Input: part model. Units: mm. Frame: model coordinates. Face numbers are marked on the shaded views. A direction names the side the tool comes from. Round coordinates to 2 decimals unless told otherwise and drop trailing zeros. Loops run counter-clockwise (first coordinate to the right, second up) from the corner with the lowest first, then second, coordinate; pieces in that order, holes last. Notation, with made-up numbers: M 38,44 L 47,44 A22 cw 47,79 Z; hole C 37,33.25 d5. An arc over 180 degrees is marked long. Use one line per item in the form item = value. Start each with the question number.
Q1. Ray query, line 1 along X through (y, z) = (0, 2.95); line 2 along X through (y, z) = (0, 1.85); line 3 along Y through (x, z) = (110, 3.9). Return the intervals inside material, ascending.
Q2. Section query C-C, the plane z = 5. Output: boundary loops of the cut face in (x, y).
Q3. Access query for the marked faces 5 and 6. Directions: +Z, -Z, +X, -X, +Y, -Y. A direction counts if a zero-diameter tool reaches every point of the face in a straight line with its end or side. Return the directions, or none.
Q4. Section query A-A, the plane y = 0. Output: boundary loops of the cut face in (x, z), and give its area (3 significant figures).
Q5. Section query D-D, the plane y = -2.25. Output: boundary loops of the cut face in (x, z), and give its area (3 significant figures).
Q6. First-contact query: P1, Ø4.5, axis at x = 120, y = 0, coming from the -Z side; P2, Ø3.5, axis at y = 0, z = 5, coming from the +X side; P3, Ø3.5, axis at x = 110, y = -0.5, coming from the +Z side; P4, Ø2, axis at x = 110, y = 0, coming from the -Z side. Flat tips, straight axial feed; report the tip coordinate or a pass-through.
Q7. Section query B-B, the plane x = 110. Output: boundary loops of the cut face in (y, z).
Q8. Mould query, pull axis Z, two halves, no side actions, for the marked faces 1, 2, 3 and 4. Classes: pulls with the +Z half, pulls with the -Z half, needs draft (parallel to the pull), parting line crosses it, or undercut.
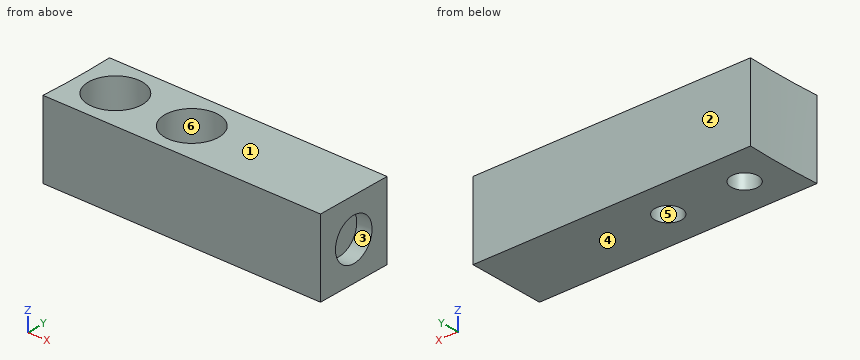
```python
from build123d import *

# Parameters (mm, degrees)
ESQUISSE1_R             = 1.75
BOSS_EXTRU_1_DEPTH      = 10
ESQUISSE2_R             = 2.75
ENL_V_MAT_EXTRU_1_DEPTH = 2
ESQUISSE3_R             = 3.5
ENL_V_MAT_EXTRU_2_DEPTH = 4


with BuildPart() as part:
    # Esquisse1 → Boss.-Extru.1 (new body)
    with BuildSketch(Plane.XY):
        with BuildLine():
            Line((104.880884817, 5), (141.2, 5))
            Line((141.2, 5), (141.2, -5))
            Line((141.2, -5), (104.880884817, -5))
            ThreePointArc((104.880884817, -5), (105, 0), (104.880884817, 5))
        make_face()
        with Locations((110, 0)):
            Circle(ESQUISSE1_R, mode=Mode.SUBTRACT)
        with Locations((120, 0)):
            Circle(ESQUISSE1_R, mode=Mode.SUBTRACT)
    extrude(amount=BOSS_EXTRU_1_DEPTH)

    # Esquisse2 → Enlèv. mat.-Extru.1 (cut)
    with BuildSketch(Plane(origin=(141.2, 0, 0), x_dir=(0, 0, -1), z_dir=(1, 0, 0))):
        with Locations((-5, 0)):
            Circle(ESQUISSE2_R)
    extrude(amount=-ENL_V_MAT_EXTRU_1_DEPTH, mode=Mode.SUBTRACT)

    # Esquisse3 → Enlèv. mat.-Extru.2 (cut)
    with BuildSketch(Plane.XY.offset(10)):
        with Locations((110, 0)):
            Circle(ESQUISSE3_R)
        with Locations((120, 0)):
            Circle(ESQUISSE3_R)
    extrude(amount=-ENL_V_MAT_EXTRU_2_DEPTH, mode=Mode.SUBTRACT)


solid = part.part
```
Results found:
q1.line_1 = 105 to 108.25, 111.75 to 118.25, 121.75 to 139.2
q1.line_2 = 105 to 108.25, 111.75 to 118.25, 121.75 to 141.2
q1.line_3 = -5 to -1.75, 1.75 to 5
q2.outline = M 104.88,-5 L 141.2,-5 L 141.2,-2.75 L 139.2,-2.75 L 139.2,2.75 L 141.2,2.75 L 141.2,5 L 104.88,5 A105 cw Z; hole C 110,0 d3.5; hole C 120,0 d3.5
q3.face_5 = +Z, -Z
q3.face_6 = +Z
q4.outline = M 105,0 L 108.25,0 L 108.25,6 L 106.5,6 L 106.5,10 L 105,10 Z; M 111.75,0 L 118.25,0 L 118.25,6 L 116.5,6 L 116.5,10 L 113.5,10 L 113.5,6 L 111.75,6 Z; M 121.75,0 L 141.2,0 L 141.2,2.25 L 139.2,2.25 L 139.2,7.75 L 141.2,7.75 L 141.2,10 L 123.5,10 L 123.5,6 L 121.75,6 Z
q4.area = 253 mm²
q5.outline = M 104.98,0 L 141.2,0 L 141.2,3.42 L 139.2,3.42 L 139.2,6.58 L 141.2,6.58 L 141.2,10 L 122.68,10 L 122.68,6 L 117.32,6 L 117.32,10 L 112.68,10 L 112.68,6 L 107.32,6 L 107.32,10 L 104.98,10 Z
q5.area = 313 mm²
q6.P1 = 0
q6.P2 = 139.2
q6.P3 = 6
q6.P4 = through
q7.outline = M -5,0 L -1.75,0 L -1.75,6 L -3.5,6 L -3.5,10 L -5,10 Z; M 1.75,0 L 5,0 L 5,10 L 3.5,10 L 3.5,6 L 1.75,6 Z
q8.face_1 = pulls with the +Z half
q8.face_2 = needs draft
q8.face_3 = undercut
q8.face_4 = pulls with the -Z half
